Here's how the part is built. I have some questions about the finished solid (model axes, mm). A direction names the side the tool comes from. Give positions to 0.01 mm unless a question says otherwise; leave off trailing zeros. Answer as CSV lines item,"result". Start each with the question number.
Item 1: For faces 1 (the flat face through (-2, 1.85, 5)), 2 (the flat face through (0, 0, 5.6)), which set-ups out of +Z, -Z, +X, -X, +Y, -Y let a thin tool reach every point of the face, with its end or its side?
Item 2: If I drill on line 1 along X through (y, z) = (1.2, 5); line 2 along Z through (x, y) = (-0.75, -0.5); line 3 along X through (y, z) = (0.7, 4.9), over which ranges is the centre line in solid material (lowest first)? Write a range as from..to.
Item 3: Will this pin go through, and if not, where does the flat tip stop? P1, Ø1.1, axis at x = 3, y = -0.5, coming from the +Z side.
Item 4: I want a section at A-A on z = 5. Give the number of separate pieces and of enclosed holes in the cut face, plus the area to 3 significant figures.
Item 5: If we mould it in two halves opening along Y, with no side actions, what happens to faces 3 (the flat face through (0, 2.25, 3)), 4 (the flat face through (2, 1.85, 5)), 5 (the flat face through (-2, 0, 5.6)), 6 (the flat face through (-2, -1.85, 5))? For each: released by +Y, released by -Y, zero draft, split by the parting line, or undercut.
from build123d import *

# Parameters (mm, degrees)
F0_W     = 9
F0_H     = 4.5
F1_DEPTH = 5.6
F2_W     = 3.7
F2_H     = 3.7
F2_R     = 1.45
F3_DEPTH = 1
F4_R     = 0.99999
F5_SIZE  = 0.5


# Not quite as in the source:
# - a fillet or chamfer is up to 0.001 mm smaller than in the source, because OpenCascade refuses the exact size


with BuildPart() as f1:
    # F0 (on Top) → F1 (new body)
    with BuildSketch(Plane.XY):
        Rectangle(F0_W, F0_H)
    extrude(amount=F1_DEPTH)

    # F2 (on face) → F3 (cut)
    with BuildSketch(Plane.XY.offset(5.6)):
        with Locations((-2.25, 0)):
            Rectangle(F2_W, F2_H)
        with Locations((-2.25, 0)):
            Circle(F2_R, mode=Mode.SUBTRACT)
        with Locations((2.25, 0)):
            Rectangle(F2_W, F2_H)
        with Locations((2.25, 0)):
            Circle(F2_R, mode=Mode.SUBTRACT)
    extrude(amount=-F3_DEPTH, mode=Mode.SUBTRACT)

    # F4 (radius 1 in the source; OpenCascade refuses exactly that, so slightly less here)
    f4_edges = [f1.edges().sort_by_distance(p)[0] for p in [
        (-3.7, 0, 5.6),
        (0.8, 0, 5.6),
    ]]
    fillet(f4_edges, radius=F4_R)

    # F5
    f5_edges = [f1.edges().sort_by_distance(p)[0] for p in [
        (4.5, 2.25, 2.8),
    ]]
    chamfer(f5_edges, length=F5_SIZE)


solid = f1.part
Result:
1,face 1,"+Z"
1,face 2,"+Z, +X, -X, +Y, -Y"
2,line 1,"-4.5..-4.1, -2.9..-1.6, -0.4..0.4, 1.6..2.9, 4.1..4.5"
2,line 2,"0..4.6"
2,line 3,"-4.5..-4.1, -3.47..-1.03, -0.4..0.4, 1.03..3.47, 4.1..4.5"
3,P1,"z = 5.6"
4,separate pieces,"3"
4,enclosed holes,"2"
4,area,"24.7 mm^2"
5,face 3,"released by +Y"
5,face 4,"undercut"
5,face 5,"zero draft"
5,face 6,"undercut"
